Read the model definition and answer for the solid it produces. Units are mm, in the model's axes. A direction names the side the tool comes from. Coordinates: 2 decimals unless noted, no trailing zeros. Write each loop counter-clockwise with the first axis right and the second up, starting at its lowest first coordinate (ties: lowest second). Pieces come first, ordered by that corner, then holes.
Item 1: Straight lines are drawn through the part: probe 1 along X at (y, z) = (39, -17.5); probe 2 along Z at (x, y) = (36, 6); probe 3 along Z at (x, y) = (-52, 37.5). For each, find the intervals that lie inside material, in ascending order.
Item 2: Determine the mould class of faces 6 (the face through (70.13, 56.82, -30.59)), 7 (the face through (0, 0, -79)), 8 (the face through (60, 64, -3)), 9 (the face through (-66.486, 29.58, -74.297)) for opening direction X: released by +X, released by -X, zero draft, split by the parting line, or undercut.
Item 3: A tool of negligible diameter and unlimited length cuts with its end or side. For faces 1 (the face through (0.73, 56.82, -77.63)), 2 (the face through (-1, 63, -4)), 3 (the face through (-1, 30, 0)), 4 (the face through (69, 62, -51)), 5 (the face through (1, 30, -80)), from which of +Z, -Z, +X, -X, +Y, -Y can it reach the whole face along a straight path? Write none if from no direction.
Item 4: Section C-C (y = 46.5) is taken. Give the vertices of the cut face in (x, z), then the cut area to 3 significant figures.
Item 5: Each of these flat-tipped pins is pushed along its axis until it touches: P1, Ø1.6, axis at x = -4.5, y = 61.5, coming from the -Z side; P2, Ø1, axis at x = 1, y = 61, coming from the +Z side; P3, Ø3, axis at y = 26, z = -70, coming from the -X side. Where does it stop, or does it pass through?
from build123d import *

# Parameters (mm, degrees)
EXTRUDE_1_DEPTH     = 60
EXTRUDE_START       = -1
EXTRUDE_2_DEPTH     = 1
CHAMFER_3_SIZE      = 2
EXTRUDE_8_DEPTH     = 2
EXTRUDE_9_DEPTH     = 30
EXTRUDE_10_DEPTH    = 60
CUT_EXTRUDE_2_DEPTH = 60.5
CUT_EXTRUDE_3_DEPTH = 30.5
CHAMFER_6_SIZE      = 0.5
FILLET_3_R          = 5
FILLET_4_R          = 0.5
FILLET_5_R          = 0.5


with BuildPart() as part:
    # Эскиз1 → Бобышка-Вытянуть1 (new body)
    with BuildSketch(Plane(origin=(0, 0, 0), x_dir=(1, 0, 0), z_dir=(0, 1, 0))):
        with BuildLine():
            Line((-72.5, 0), (72.5, 0))
            Line((72.5, 0), (72.5, 60))
            ThreePointArc((72.5, 60), (66.642135624, 74.142135624), (52.5, 80))
            Line((52.5, 80), (-52.5, 80))
            ThreePointArc((-52.5, 80), (-66.642135624, 74.142135624), (-72.5, 60))
            Line((-72.5, 60), (-72.5, 0))
        make_face()
        with BuildLine():
            Line((-70.5, 2), (70.5, 2))
            Line((70.5, 2), (70.5, 60))
            ThreePointArc((70.5, 60), (65.227922061, 72.727922061), (52.5, 78))
            Line((52.5, 78), (-52.5, 78))
            ThreePointArc((-52.5, 78), (-65.227922061, 72.727922061), (-70.5, 60))
            Line((-70.5, 60), (-70.5, 2))
        make_face(mode=Mode.SUBTRACT)
    extrude(amount=EXTRUDE_1_DEPTH)

    # Эскиз2 → Бобышка-Вытянуть2 (add)
    with BuildSketch(Plane(origin=(0, 60, 0), x_dir=(1, 0, 0), z_dir=(0, 1, 0)).offset(EXTRUDE_START)):
        with BuildLine():
            Line((-72.5, 60), (-72.5, 0))
            Line((-72.5, 0), (72.5, 0))
            Line((72.5, 0), (72.5, 60))
            ThreePointArc((72.5, 60), (66.642135624, 74.142135624), (52.5, 80))
            Line((52.5, 80), (-52.5, 80))
            ThreePointArc((-52.5, 80), (-66.642135624, 74.142135624), (-72.5, 60))
        make_face()
        with BuildLine():
            Line((-68.5, 60), (-68.5, 4))
            Line((-68.5, 4), (68.5, 4))
            Line((68.5, 4), (68.5, 60))
            ThreePointArc((68.5, 60), (63.813708499, 71.313708499), (52.5, 76))
            Line((52.5, 76), (-52.5, 76))
            ThreePointArc((-52.5, 76), (-63.813708499, 71.313708499), (-68.5, 60))
        make_face(mode=Mode.SUBTRACT)
    extrude(amount=EXTRUDE_2_DEPTH)

    # Фаска3
    chamfer_3_edges = [part.edges().sort_by_distance(p)[0] for p in [
        (-65.227922061, 59, -72.727922061),
        (-70.5, 59, -31),
        (0, 59, -2),
        (70.5, 59, -31),
        (65.227922061, 59, -72.727922061),
        (0, 59, -78),
    ]]
    chamfer(chamfer_3_edges, length=CHAMFER_3_SIZE - 0.0001)  # a hair under: the kernel refuses the full size

    # Эскиз11 → Бобышка-Вытянуть8 (add)
    with BuildSketch(Plane(origin=(0, 60, 0), x_dir=(1, 0, 0), z_dir=(0, 1, 0))):
        with BuildLine():
            Line((70.25, 2.25), (70.25, 60))
            ThreePointArc((70.25, 60), (65.051145366, 72.551145366), (52.5, 77.75))
            Line((52.5, 77.75), (-52.5, 77.75))
            ThreePointArc((-52.5, 77.75), (-65.051145366, 72.551145366), (-70.25, 60))
            Line((-70.25, 60), (-70.25, 2.25))
            Line((-70.25, 2.25), (70.25, 2.25))
        make_face()
        with BuildLine():
            Line((68.5, 4), (68.5, 60))
            ThreePointArc((68.5, 60), (63.813708499, 71.313708499), (52.5, 76))
            Line((52.5, 76), (-52.5, 76))
            ThreePointArc((-52.5, 76), (-63.813708499, 71.313708499), (-68.5, 60))
            Line((-68.5, 60), (-68.5, 4))
            Line((-68.5, 4), (68.5, 4))
        make_face(mode=Mode.SUBTRACT)
    extrude(amount=EXTRUDE_8_DEPTH)

    # Эскиз12 → Бобышка-Вытянуть9 (add, symmetric)
    with BuildSketch(Plane(origin=(0, 0, 0), x_dir=(0, 0, -1), z_dir=(1, 0, 0))):
        Polygon((76, 62), (76, 66.7), (77.75, 66.7), (79.45, 65), (77.75, 63.3), (77.75, 62), align=None)
    extrude(amount=EXTRUDE_9_DEPTH, both=True)

    # Эскиз13 → Бобышка-Вытянуть10 (add, symmetric)
    with BuildSketch(Plane(origin=(0, 0, 0), x_dir=(0, 0, -1), z_dir=(1, 0, 0))):
        Polygon((2.25, 62), (2.25, 63.3), (0.55, 65), (2.25, 66.7), (4, 66.7), (4, 62), align=None)
    extrude(amount=EXTRUDE_10_DEPTH, both=True)

    # Эскиз15 → Вырез-Вытянуть2 (cut, symmetric)
    with BuildSketch(Plane(origin=(0, 0, 0), x_dir=(0, 0, -1), z_dir=(1, 0, 0))):
        Polygon((2, 3.5), (2, 6.5), (0.5, 5), align=None)
    extrude(amount=CUT_EXTRUDE_2_DEPTH, both=True, mode=Mode.SUBTRACT)

    # Эскиз16 → Вырез-Вытянуть3 (cut, symmetric)
    with BuildSketch(Plane(origin=(0, 0, 0), x_dir=(0, 0, -1), z_dir=(1, 0, 0))):
        Polygon((78, 3.5), (78, 6.5), (79.5, 5), align=None)
    extrude(amount=CUT_EXTRUDE_3_DEPTH, both=True, mode=Mode.SUBTRACT)

    # Фаска6
    chamfer_6_edges = [part.edges().sort_by_distance(p)[0] for p in [
        (-70.5, 0, -31),
        (0, 0, -2),
        (70.5, 0, -31),
        (65.227922061, 0, -72.727922061),
        (0, 0, -78),
        (-65.227922061, 0, -72.727922061),
    ]]
    chamfer(chamfer_6_edges, length=CHAMFER_6_SIZE)

    # Скругление3
    fillet_3_edges = [part.edges().sort_by_distance(p)[0] for p in [
        (70.5, 57.0001, -31),
        (65.227922061, 57.0001, -72.727922061),
        (0, 57.0001, -78),
        (-65.227922061, 57.0001, -72.727922061),
        (0, 57.0001, -2),
        (-70.5, 57.0001, -31),
    ]]
    fillet(fillet_3_edges, radius=FILLET_3_R)

    # Скругление4
    fillet_4_edges = [part.edges().sort_by_distance(p)[0] for p in [
        (0, 5, -0.5),
        (0, 5, -79.5),
    ]]
    fillet(fillet_4_edges, radius=FILLET_4_R)

    # Скругление5
    fillet_5_edges = [part.edges().sort_by_distance(p)[0] for p in [
        (0, 65, -79.45),
        (0, 65, -0.55),
    ]]
    fillet(fillet_5_edges, radius=FILLET_5_R)


solid = part.part
Established:
1. probe 1: x = -72.5 to -70.5, 70.5 to 72.5
1. probe 2: z = -80 to -78, -1.5 to 0
1. probe 3: z = -80 to -78, -2 to 0
2. face 6: undercut
2. face 7: zero draft
2. face 8: released by +X
2. face 9: released by -X
3. face 1: -Y
3. face 2: +Y, -Y
3. face 3: +Z, +X, -X, +Y, -Y
3. face 4: -Z, +X, +Y
3. face 5: -Z, +X, -X, +Y, -Y
4. outline: (-72.5, -60) arc R20 ccw to (-52.5, -80) - (52.5, -80) arc R20 ccw to (72.5, -60) - (72.5, 0) - (-72.5, 0) - close; hole (-70.5, -60) arc R18 ccw to (-52.5, -78) - (52.5, -78) arc R18 ccw to (70.5, -60) - (70.5, -2) - (-70.5, -2) - close
4. area: 851 mm2
5. P1: stops at z = -77.75
5. P2: stops at z = -2.25
5. P3: stops at x = -70.6
